Check sheet for the modelled part. Datum: model origin and axes. Units: mm. A direction names the side the tool comes from. Round coordinates to 2 decimals unless told otherwise and drop trailing zeros. Order: outer loops, then holes, each group sorted by start corner. A loop starts at its lowest first (then second) coordinate and runs counter-clockwise, first axis right, second up. Notation, with made-up numbers: (-22.5, 76.5) -> (12.5, 76.5) arc R28 cw to (12.5, 106.5) -> close; hole circle Ø6 at (14, 35). An arc over 180 degrees is marked (long way). Answer in a Markdown table with one row per item. Add a question column.
1. Sectioned sample at B-B, the plane y = 6.35. Record the boundary of the cut face in (x, z) (1 decimal).
2. Draft check along Y on faces 1 (the cylindrical face through (-1.57, 78.18, -13.6)), 2 (the flat face through (-2, 237.49, -7)), 3 (the flat face through (-2, 0, -7)), 4 (the flat face through (-17, 117, -3.175)). Enter one of: +Y half, -Y half, draft (parallel to the pull), parting line (faces both ways), or undercut.
3. Sectioned sample at D-D, the plane y = 112. Record the boundary of the cut face in (x, z) (3 decimals), then the cut area to 3 significant figures.
4. Sectioned sample at A-A, the plane x = -12.7. Record the boundary of the cut face in (y, z) (3 decimals).
5. Depth check by flat-ended pin: P1, Ø5, axis at x = -10.5, z = -7, coming from the -Y side; P2, Ø1, axis at x = -11.5, y = 60, coming from the -Z side (3 decimals); P3, Ø6.5, axis at y = 154.5, z = -12.5, coming from the -X side (3 decimals). Enter the tip coordinate at first touch or a pass-through.
6. Access from +Z, -Z, +X, -X, +Y, -Y to the whole of each face (thin tool, end or side, straight path). Record for faces 5 (the cylindrical face through (-1.565, 6.49, -11.116)), 6 (the flat face through (-3.175, 117, -14)).
7. Sectioned sample at C-C, the plane z = -8. Record the boundary of the cut face in (x, y) (3 decimals), then the cut area to 3 significant figures.
8. Material ranges on L1, parallel to Y at x = -12.7, z = -2.05 (3 decimals); L2, parallel to Y at x = -11.25, z = -2; L3, parallel to Z at x = -0.9, y = 231.14, recorded low to high. Write a range as from..to.
Autodesk Inventor part; units mm, degrees
ref_plane "YZ Plane" through (0, 0, 0) normal (1, 0, 0) x (0, 1, 0)
ref_plane "XZ Plane" through (0, 0, 0) normal (0, 1, 0) x (-1, 0, 0)
ref_plane "XY Plane" through (0, 0, 0) normal (0, 0, 1) x (1, 0, 0)
sketch "Sketch1" plane through (0, 0, 0) normal (0, 1, 0) x (-1, 0, 0)
  line L0 (0, 0) -> (0, -25.4)
  line L1 (0, -25.4) -> (3.175, -25.4)
  line L2 (3.175, -25.4) -> (3.175, -3.175)
  line L3 (3.175, -3.175) -> (25.4, -3.175)
  line L4 (25.4, -3.175) -> (25.4, 0)
  line L5 (25.4, 0) -> (0, 0)
  dimension "d0" = 25.4
  dimension "d1" = 3.175
  dimension "d2" = 22.225
  dimension "d3" = 22.225
extrude "Extrusion1" add sketch "Sketch1" along normal blind 237.49
sketch "Sketch4" plane through (0, 0, 0) normal (1, 0, 0) x (0, 0, -1)
  line L0 (25.4, 0) -> (3.175, 0)
  line L1 (25.4, 237.49) -> (3.175, 237.49)
  circle A0 centre (14.2875, 231.14) radius 3.175
  circle A1 centre (14.2875, 6.35) radius 3.175
  circle A2 centre (14.2875, 156.21) radius 3.175
  circle A3 centre (14.2875, 81.28) radius 3.175
  point P0 (0, 0)
  dimension "d23" = 6.35
  dimension "d26" = 6.35
  dimension "d27" = 6.35
extrude "Extrusion4" cut sketch "Sketch4" against normal blind 237.49
sketch "Sketch5" plane through (-25.4, 0, 0) normal (0, 0, 1) x (1, 0, 0)
  line L0 (0, 0) -> (25.4, 0)
  line L1 (22.225, 237.49) -> (0, 237.49)
  circle A0 centre (12.7, 212.09) radius 3.175
  circle A1 centre (12.7, 118.745) radius 3.175
  circle A2 centre (12.7, 25.4) radius 3.175
  dimension "d32" = 6.35
  dimension "d33" = 6.35
  dimension "d34" = 6.35
extrude "Extrusion5" cut sketch "Sketch5" against normal blind 237.49
properties part number "Cylinder Bracket"
Answer key:
| question | item | result |
|---|---|---|
| 1 | outline | (-25.4, -3.2) -> (-3.2, -3.2) -> (-3.2, -11.1) -> (0, -11.1) -> (0, 0) -> (-25.4, 0) -> close; (-3.2, -25.4) -> (0, -25.4) -> (0, -17.5) -> (-3.2, -17.5) -> close |
| 2 | face 1 | undercut |
| 2 | face 2 | +Y half |
| 2 | face 3 | -Y half |
| 2 | face 4 | draft |
| 3 | outline | (-25.4, -3.175) -> (-3.175, -3.175) -> (-3.175, -25.4) -> (0, -25.4) -> (0, 0) -> (-25.4, 0) -> close |
| 3 | area | 151 mm² |
| 4 | outline | (0, -3.175) -> (22.225, -3.175) -> (22.225, 0) -> (0, 0) -> close; (28.575, -3.175) -> (115.57, -3.175) -> (115.57, 0) -> (28.575, 0) -> close; (121.92, -3.175) -> (208.915, -3.175) -> (208.915, 0) -> (121.92, 0) -> close; (215.265, -3.175) -> (237.49, -3.175) -> (237.49, 0) -> (215.265, 0) -> close |
| 5 | P1 | passes through |
| 5 | P2 | stops at z = -3.175 |
| 5 | P3 | stops at x = -3.175 |
| 6 | face 5 | +X, -X |
| 6 | face 6 | -Z, -X, +Y, -Y |
| 7 | outline | (-3.175, 0) -> (0, 0) -> (0, 237.49) -> (-3.175, 237.49) -> close |
| 7 | area | 754 mm² |
| 8 | L1 | y = 0..22.225, 28.575..115.57, 121.92..208.915, 215.265..237.49 |
| 8 | L2 | y = 0..22.58, 28.22..115.92, 121.57..209.27, 214.91..237.49 |
| 8 | L3 | z = -25.4..-17.46, -11.11..0 |
